```python
from build123d import *

# Parameters (mm, degrees)
BOSS_EXTRUDE1_DEPTH = 7.55
SKETCH4_R           = 3
SKETCH4_R_2         = 7
BOSS_EXTRUDE2_DEPTH = 6.01
SKETCH5_R           = 3.25
SKETCH5_R_2         = 2.25
CUT_EXTRUDE1_DEPTH  = 0.5
BOSS_EXTRUDE3_DEPTH = 1.15
BOSS_EXTRUDE4_DEPTH = 1.5
BOSS_EXTRUDE5_DEPTH = 1.5
BOSS_EXTRUDE6_DEPTH = 1.5
BOSS_EXTRUDE7_DEPTH = 1.5
SKETCH15_R          = 0.75
SKETCH15_R_2        = 0.282518913
CUT_EXTRUDE2_DEPTH  = 105.40765585
SKETCH16_R          = 1
SKETCH16_R_2        = 0.902700303
SKETCH16_R_3        = 0.840140681
CUT_EXTRUDE3_DEPTH  = 1.5


with BuildPart() as part:
    # Sketch2 → Boss-Extrude1 (new body)
    with BuildSketch(Plane.XY):
        with BuildLine():
            Line((-27.75, 73.75), (27.75, 73.75))
            ThreePointArc((27.75, 73.75), (33.406854249, 71.406854249), (35.75, 65.75))
            Line((35.75, 65.75), (35.75, -65.75))
            ThreePointArc((35.75, -65.75), (33.406854249, -71.406854249), (27.75, -73.75))
            Line((27.75, -73.75), (-27.75, -73.75))
            ThreePointArc((-27.75, -73.75), (-33.406854249, -71.406854249), (-35.75, -65.75))
            Line((-35.75, -65.75), (-35.75, 65.75))
            ThreePointArc((-35.75, 65.75), (-33.406854249, 71.406854249), (-27.75, 73.75))
        make_face()
    extrude(amount=BOSS_EXTRUDE1_DEPTH)

    # Sketch4 → Boss-Extrude2 (add)
    with BuildSketch(Plane.XY.offset(7.55)):
        with BuildLine():
            ThreePointArc((-1.025851878, 68.342271784), (2.509682028, 66.87780569), (3.974148122, 63.342271784))
            Line((3.974148122, 63.342271784), (3.974148122, 35.132271784))
            ThreePointArc((3.974148122, 35.132271784), (2.509682028, 31.596737878), (-1.025851878, 30.132271784))
            Line((-1.025851878, 30.132271784), (-27.755851878, 30.132271784))
            ThreePointArc((-27.755851878, 30.132271784), (-31.291385784, 31.596737878), (-32.755851878, 35.132271784))
            Line((-32.755851878, 35.132271784), (-32.755851878, 63.342271784))
            ThreePointArc((-32.755851878, 63.342271784), (-31.291385784, 66.87780569), (-27.755851878, 68.342271784))
            Line((-27.755851878, 68.342271784), (-1.025851878, 68.342271784))
        make_face()
        with Locations(Location((-5.550757153, 63.342271784, 0), (0, 0, 180))):
            Circle(SKETCH4_R, mode=Mode.SUBTRACT)
        with Locations(Location((-5.550757153, 49.237271784, 0), (0, 0, 180))):
            Circle(SKETCH4_R_2, mode=Mode.SUBTRACT)
        with Locations(Location((-25.170144884, 38.02363754, 0), (0, 0, 180))):
            Circle(SKETCH4_R_2, mode=Mode.SUBTRACT)
        with Locations(Location((-25.170144884, 60.450906027, 0), (0, 0, 180))):
            Circle(SKETCH4_R_2, mode=Mode.SUBTRACT)
    extrude(amount=BOSS_EXTRUDE2_DEPTH)

    # Sketch5 → Cut-Extrude1 (cut)
    # profile 1 of 2: a face of its own
    with BuildSketch(Plane(origin=(0, 0, 0), x_dir=(-1, 0, 0), z_dir=(0, 0, -1))):
        with Locations((8.017760332, 66.917461234)):
            Circle(SKETCH5_R)
        with Locations((8.017760332, 66.917461234)):
            Circle(SKETCH5_R_2, mode=Mode.SUBTRACT)
    # profile 2 of 2: a face of its own
    with BuildSketch(Plane(origin=(0, 0, 0), x_dir=(-1, 0, 0), z_dir=(0, 0, -1))):
        with BuildLine():
            Line((0.126908454, 64.039290859), (-6.373091546, 64.039290859))
            ThreePointArc((-6.373091546, 64.039290859), (-9.251261922, 66.917461234), (-6.373091546, 69.79563161))
            Line((-6.373091546, 69.79563161), (0.126908454, 69.79563161))
            ThreePointArc((0.126908454, 69.79563161), (3.00507883, 66.917461234), (0.126908454, 64.039290859))
        make_face()
        with Locations((0.126908454, 66.917461234)):
            Circle(SKETCH5_R_2, mode=Mode.SUBTRACT)
        with Locations((-6.373091546, 66.917461234)):
            Circle(SKETCH5_R_2, mode=Mode.SUBTRACT)
    extrude(amount=-CUT_EXTRUDE1_DEPTH, mode=Mode.SUBTRACT)

    # Sketch6 → Boss-Extrude3 (add)
    with BuildSketch(Plane.ZY.offset(35.75)):
        with BuildLine():
            Line((1.817009034, 15.75), (1.817009034, 31.75))
            ThreePointArc((1.817009034, 31.75), (3.317009034, 33.25), (4.817009034, 31.75))
            Line((4.817009034, 31.75), (4.817009034, 15.75))
            ThreePointArc((4.817009034, 15.75), (3.317009034, 14.25), (1.817009034, 15.75))
        make_face()
        with BuildLine():
            Line((1.817009034, -31.25), (1.817009034, -11.25))
            ThreePointArc((1.817009034, -11.25), (3.317009034, -9.75), (4.817009034, -11.25))
            Line((4.817009034, -11.25), (4.817009034, -31.25))
            ThreePointArc((4.817009034, -31.25), (3.317009034, -32.75), (1.817009034, -31.25))
        make_face()
    extrude(amount=BOSS_EXTRUDE3_DEPTH)

    # Sketch11 → Boss-Extrude4 (add)
    with BuildSketch(Plane(origin=(35.75, 0, 0), x_dir=(0, 0, -1), z_dir=(1, 0, 0))):
        with BuildLine():
            Line((-2.110967664, 47.91857343), (-2.110967664, 41.91857343))
            ThreePointArc((-2.110967664, 41.91857343), (-3.620147118, 40.409393977), (-5.129326571, 41.91857343))
            Line((-5.129326571, 41.91857343), (-5.129326571, 47.91857343))
            ThreePointArc((-5.129326571, 47.91857343), (-3.620147118, 49.427752884), (-2.110967664, 47.91857343))
        make_face()
    extrude(amount=BOSS_EXTRUDE4_DEPTH)

    # Sketch12 → Boss-Extrude5 (add)
    with BuildSketch(Plane(origin=(35.75, 0, 0), x_dir=(0, 0, -1), z_dir=(1, 0, 0))):
        with BuildLine():
            Line((-2.275343981, 34.931061823), (-2.275343981, 22.931061823))
            ThreePointArc((-2.275343981, 22.931061823), (-3.375343981, 21.831061823), (-4.475343981, 22.931061823))
            Line((-4.475343981, 22.931061823), (-4.475343981, 34.931061823))
            ThreePointArc((-4.475343981, 34.931061823), (-3.375343981, 36.031061823), (-2.275343981, 34.931061823))
        make_face()
    extrude(amount=BOSS_EXTRUDE5_DEPTH)

    # Sketch13 → Boss-Extrude6 (add)
    with BuildSketch(Plane(origin=(35.75, 0, 0), x_dir=(0, 0, -1), z_dir=(1, 0, 0))):
        with BuildLine():
            Line((-2.160495945, 19.909535664), (-2.160495945, 7.909535664))
            ThreePointArc((-2.160495945, 7.909535664), (-3.260495945, 6.809535664), (-4.360495945, 7.909535664))
            Line((-4.360495945, 7.909535664), (-4.360495945, 19.909535664))
            ThreePointArc((-4.360495945, 19.909535664), (-3.260495945, 21.009535664), (-2.160495945, 19.909535664))
        make_face()
    extrude(amount=BOSS_EXTRUDE6_DEPTH)

    # Sketch14 → Boss-Extrude7 (add)
    with BuildSketch(Plane(origin=(35.75, 0, 0), x_dir=(0, 0, -1), z_dir=(1, 0, 0))):
        with BuildLine():
            Line((-2.217009034, -11.25), (-2.217009034, -25.25))
            ThreePointArc((-2.217009034, -25.25), (-3.317009034, -26.35), (-4.417009034, -25.25))
            Line((-4.417009034, -25.25), (-4.417009034, -11.25))
            ThreePointArc((-4.417009034, -11.25), (-3.317009034, -10.15), (-2.217009034, -11.25))
        make_face()
    extrude(amount=BOSS_EXTRUDE7_DEPTH)

    # Sketch15 → Cut-Extrude2 (cut, through all)
    with BuildSketch(Plane(origin=(35.75, 0, 0), x_dir=(0, 0, -1), z_dir=(1, 0, 0))):
        with Locations(Location((-3.338668138, -22.921678058, 0), (0, 0, 90))):
            Circle(SKETCH15_R)
        with Locations(Location((-3.338668138, -22.921678058, 0), (0, 0, 90))):
            Circle(SKETCH15_R_2, mode=Mode.SUBTRACT)
    extrude(amount=CUT_EXTRUDE2_DEPTH, mode=Mode.SUBTRACT)

    # Sketch16 → Cut-Extrude3 (cut)
    # profile 1 of 13: a face of its own
    with BuildSketch(Plane.XZ.offset(73.75)):
        with Locations(Location((-6.64408172, 2.903732575, 0), (0, 0, 270))):
            Circle(SKETCH16_R)
        with Locations(Location((-6.64408172, 2.887582834, 0), (0, 0, 270))):
            Circle(SKETCH16_R_2, mode=Mode.SUBTRACT)
    # profile 2 of 13: a face of its own
    with BuildSketch(Plane.XZ.offset(73.75)):
        with Locations(Location((5.180713546, 2.903732575, 0), (0, 0, 270))):
            Circle(SKETCH16_R)
        with Locations(Location((5.180713546, 2.903732575, 0), (0, 0, 270))):
            Circle(SKETCH16_R_3, mode=Mode.SUBTRACT)
    # profile 3 of 13: a face of its own
    with BuildSketch(Plane.XZ.offset(73.75)):
        with Locations(Location((-12.086230414, 2.887582834, 0), (0, 0, 270))):
            Circle(SKETCH16_R)
    # profile 4 of 13: a face of its own
    with BuildSketch(Plane.XZ.offset(73.75)):
        with Locations(Location((-15.086230414, 2.887582834, 0), (0, 0, 270))):
            Circle(SKETCH16_R)
    # profile 5 of 13: a face of its own
    with BuildSketch(Plane.XZ.offset(73.75)):
        with Locations(Location((-18.086230414, 2.887582834, 0), (0, 0, 270))):
            Circle(SKETCH16_R)
    # profile 6 of 13: a face of its own
    with BuildSketch(Plane.XZ.offset(73.75)):
        with Locations(Location((-21.086230414, 2.887582834, 0), (0, 0, 270))):
            Circle(SKETCH16_R)
    # profile 7 of 13: a face of its own
    with BuildSketch(Plane.XZ.offset(73.75)):
        with Locations(Location((24.787493313, 2.903732575, 0), (0, 0, 270))):
            Circle(SKETCH16_R)
    # profile 8 of 13: a face of its own
    with BuildSketch(Plane.XZ.offset(73.75)):
        with Locations(Location((21.787493313, 2.903732575, 0), (0, 0, 270))):
            Circle(SKETCH16_R)
    # profile 9 of 13: a face of its own
    with BuildSketch(Plane.XZ.offset(73.75)):
        with Locations(Location((18.787493313, 2.903732575, 0), (0, 0, 270))):
            Circle(SKETCH16_R)
    # profile 10 of 13: a face of its own
    with BuildSketch(Plane.XZ.offset(73.75)):
        with Locations(Location((15.787493313, 2.903732575, 0), (0, 0, 270))):
            Circle(SKETCH16_R)
    # profile 11 of 13: a face of its own
    with BuildSketch(Plane.XZ.offset(73.75)):
        with Locations(Location((12.787493313, 2.903732575, 0), (0, 0, 270))):
            Circle(SKETCH16_R)
    # profile 12 of 13: a face of its own
    with BuildSketch(Plane.XZ.offset(73.75)):
        with Locations(Location((9.787493313, 2.903732575, 0), (0, 0, 270))):
            Circle(SKETCH16_R)
    # profile 13 of 13: a face of its own
    with BuildSketch(Plane.XZ.offset(73.75)):
        Polygon((-3.776371679, 3.343279725), (2.223628321, 3.343279725), (3.223628321, 2.343279725), (-4.776371679, 2.343279725), align=None)
    extrude(amount=-CUT_EXTRUDE3_DEPTH, mode=Mode.SUBTRACT)


solid = part.part
```
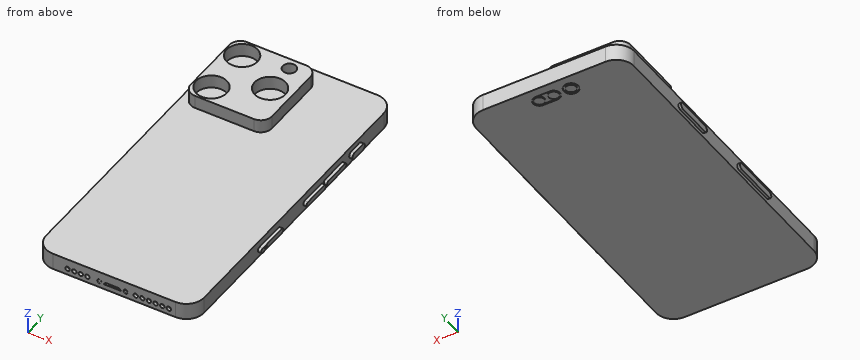
Could you check a few things on this model? Use its own coordinates, in mm. Round coordinates to 2 decimals unless told otherwise and drop trailing zeros. Write each loop counter-clockwise with the first axis right and the second up, starting at its lowest first coordinate (ties: lowest second). Pieces come first, ordered by that corner, then holes. Notation, with made-up numbers: M 53,-5 L 106,-5 A18 cw 106,11 Z; hole C -23,78.5 d6. An arc over 180 degrees is marked long. Write each question's results on one line, items separated by ' | '. Start each with the question number.
1. Imagine slicing it at A-A on y = -1. List the corners of the cut face in (x, z) for me, and give its area (3 significant figures).
2. I'm going to push flat-ended pins straight in: pin 1 Ø1.8 at (x, z) = (15.79, 2.9) entering from -Y; pin 2 Ø1.5 at (y, z) = (-37.5, 5) entering from +X; pin 3 Ø0.9 at (x, y) = (-36.5, -22) entering from +Z. Where does each tip first touch, or does it pass through?
3. I need wall thicknesses on L1, parallel to Z at x = 7, y = -5; L2, parallel to X at y = -20.5, z = 7.25; L3, parallel to Y at x = -13, z = 10.5. Which ranges of each line are inside material? Lowest first, please. Write a range as from..to.
Result sheet:
1) outline: M -35.75,0 L 35.75,0 L 35.75,7.55 L -35.75,7.55 Z | area: 540 mm^2
2) pin 1: stops at y = -72.25 | pin 2: stops at x = 35.75 | pin 3: stops at z = 4.82
3) L1: z = 0..7.55 | L2: x = -35.75..35.75 | L3: y = 30.13..68.34
